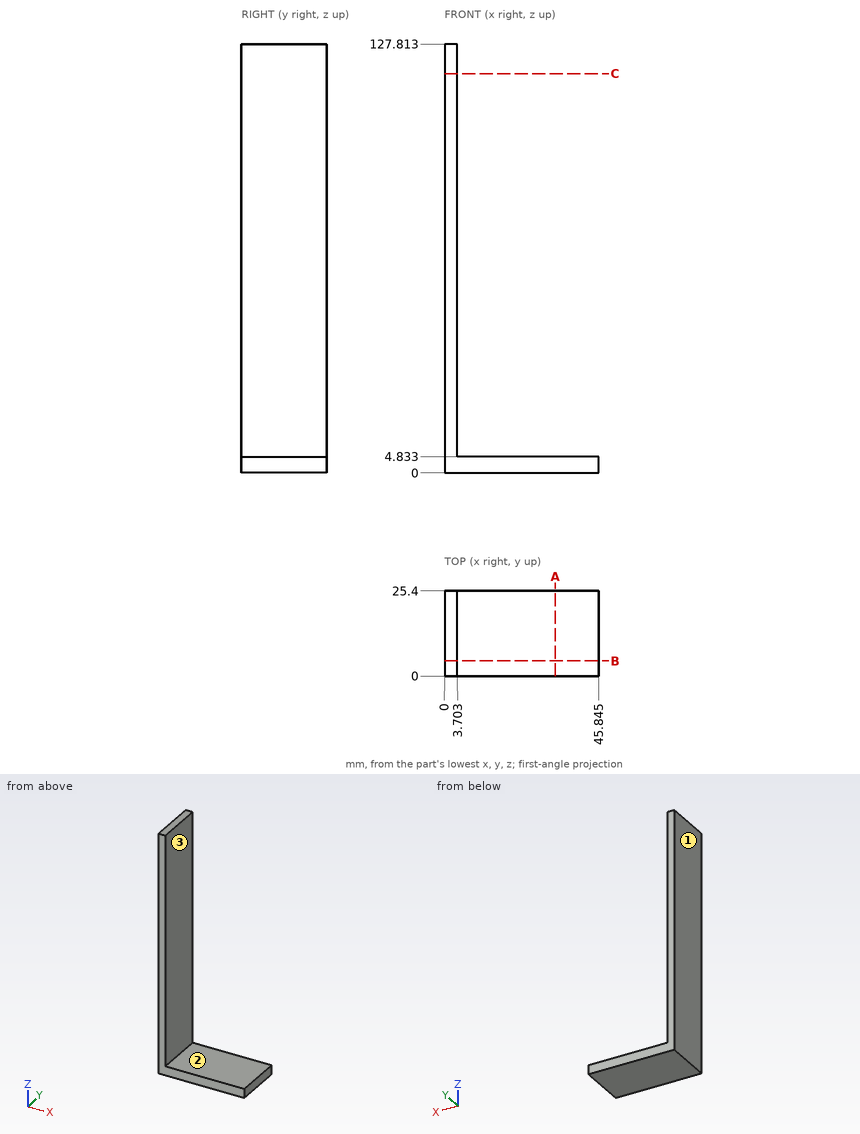
Here's the drawing with two shaded views (mm, measured from the low corner). I have some questions. Coordinates: 2 decimals unless noted, no trailing zeros. Loops run counter-clockwise (first coordinate to the right, second up) from the corner with the lowest first, then second, coordinate; pieces in that order, holes last. Notation, with made-up numbers: (11.25, -24) -> (18.25, -24) arc R15 ccw to (18.25, -2) -> close; hole circle Ø11 at (-8.75, 24). An arc over 180 degrees is marked (long way). Answer in a Markdown table with one row per item.
(1) Will these pins go through, and if not, where does the flat tip stop? pin 1 Ø1.5 at (y, z) = (7, 107.5) entering from -X; pin 2 Ø2 at (y, z) = (3.5, 41.5) entering from +X; pin 3 Ø1.5 at (x, y) = (33.5, 20) entering from +Z.
Results found:
| item | result |
|---|---|
| pin 1 | stops at x = 0 |
| pin 2 | stops at x = 3.7 |
| pin 3 | stops at z = 4.83 |
(2) Imagine slicing it at A-A (x = 33). List the corners of the cut face in (y, z) for me, plus the area to 3 significant figures.
Results found:
| item | result |
|---|---|
| outline | (0, 0) -> (25.4, 0) -> (25.4, 4.83) -> (0, 4.83) -> close |
| area | 123 mm^2 |
(3) Imagine slicing it at B-B (y = 4.5). List the corners of the cut face in (x, z) for me (1 decimal).
Results found:
| item | result |
|---|---|
| outline | (0, 0) -> (45.8, 0) -> (45.8, 4.8) -> (3.7, 4.8) -> (3.7, 127.8) -> (0, 127.8) -> close |
(4) Imagine slicing it at C-C (z = 119). List the corners of the cut face in (x, y) for me.
Results found:
| item | result |
|---|---|
| outline | (0, 0) -> (3.7, 0) -> (3.7, 25.4) -> (0, 25.4) -> close |
(5) Thinking about a two-plate mould opening in X: for the marked faces 1, 2 and 3, which applies, released by +X, released by -X, zero draft, split by the parting line, or undercut?
Results found:
| item | result |
|---|---|
| face 1 | released by -X |
| face 2 | zero draft |
| face 3 | released by +X |
(6) If I drill on probe 1 along Z at (x, y) = (16.5, 16.5); probe 2 along X at (y, z) = (19.25, 54), over which ranges is the centre line in solid material (lowest first)?
Results found:
| item | result |
|---|---|
| probe 1 | z = 0 to 4.83 |
| probe 2 | x = 0 to 3.7 |
